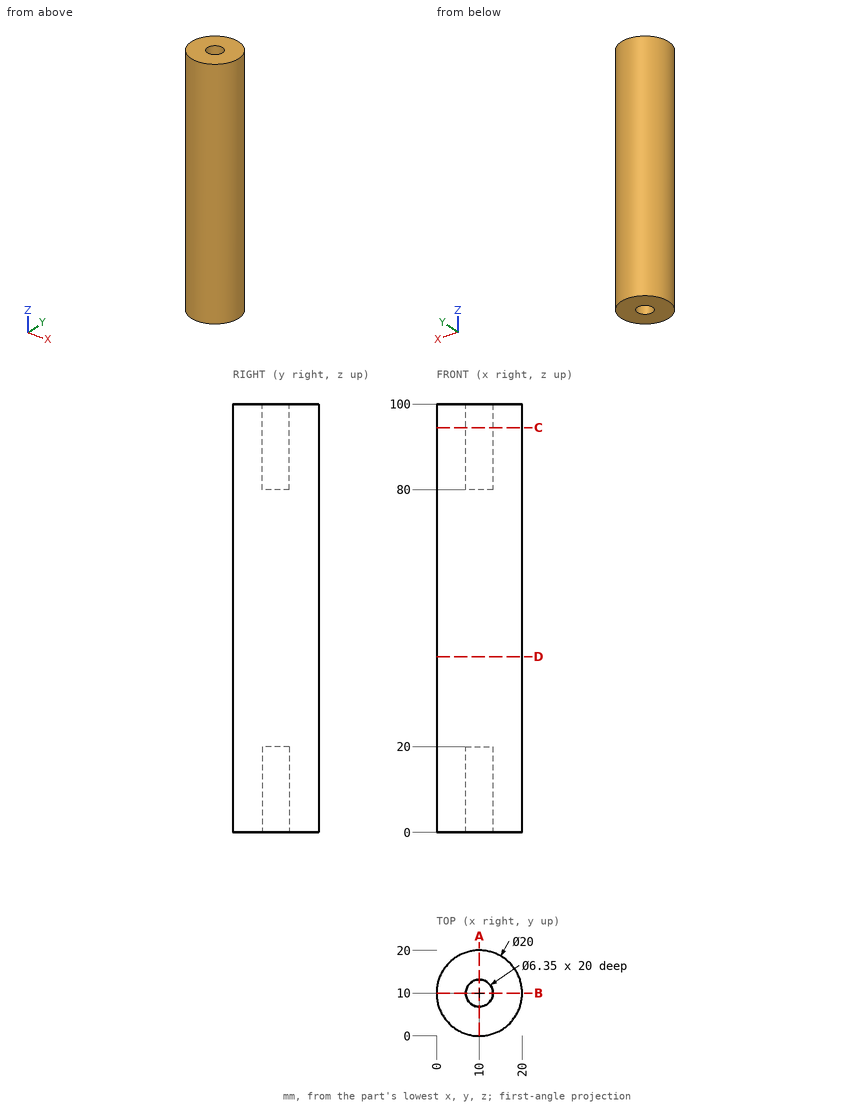
For this review, use the dimensioned drawing (mm, ordinates from the lowest corner) and the shaded views. Coordinates: 2 decimals unless noted, no trailing zeros. Loops run counter-clockwise (first coordinate to the right, second up) from the corner with the lowest first, then second, coordinate; pieces in that order, holes last. Notation, with made-up numbers: (17.25, 35) -> (53.25, 35) arc R10 ccw to (53.25, 45) -> close; hole circle Ø3 at (55, 12). An arc over 180 degrees is marked (long way). Use a Markdown table: item, result. Add a question column.
1. To check wall thickness, follow line 1 (Y direction, x = 10, z = 89) (3 decimals); line 2 (X direction, y = 12.75, z = 87.5); line 3 (Y direction, x = 6, z = 46). State the ranges of each line that lie inside material, in increasing order.
2. Add section A-A on x = 10. Write out the cut boundary in (y, z) (3 decimals), plus the area to 3 significant figures.
3. Clearance check with flat-ended pins moving along their axes: pin 1 Ø1.5 at (x, z) = (9, 80) entering from +Y; pin 2 Ø6 at (x, z) = (6, 82) entering from -Y; pin 3 Ø6 at (x, z) = (3.5, 86.5) entering from -Y. State where each tip first meets the part, or that it passes through.
4. Add section C-C on z = 94.5. Write out the cut boundary in (x, y) (3 decimals).
5. Add section D-D on z = 41. Write out the cut boundary in (x, y).
Returned:
| question | item | result |
|---|---|---|
| 1 | line 1 | y = 0 to 6.825, 13.175 to 20 |
| 1 | line 2 | x = 0.39 to 8.41, 11.59 to 19.61 |
| 1 | line 3 | y = 0.83 to 19.17 |
| 2 | outline | (0, 0) -> (6.825, 0) -> (6.825, 20) -> (13.175, 20) -> (13.175, 0) -> (20, 0) -> (20, 100) -> (13.175, 100) -> (13.175, 80) -> (6.825, 80) -> (6.825, 100) -> (0, 100) -> close |
| 2 | area | 1,750 mm² |
| 3 | pin 1 | stops at y = 20 |
| 3 | pin 2 | stops at y = 0.05 |
| 3 | pin 3 | stops at y = 0.63 |
| 4 | outline | circle Ø20 at (10, 10); hole circle Ø6.35 at (10, 10) |
| 5 | outline | circle Ø20 at (10, 10) |
